Autodesk Inventor part; units mm, degrees
ref_plane "YZ Plane" through (0, 0, 0) normal (1, 0, 0) x (0, 1, 0)
ref_plane "XZ Plane" through (0, 0, 0) normal (0, 1, 0) x (-1, 0, 0)
ref_plane "XY Plane" through (0, 0, 0) normal (0, 0, 1) x (1, 0, 0)
sketch "Esquisse1" plane through (0, 0, 0) normal (1, 0, 0) x (0, 1, 0)
  line L0 (615.5373, -142.1522) -> (811.8285, -142.1522) construction
  line L1 (811.8285, -142.1522) -> (811.8285, -230.5611) construction
  line L2 (811.8285, -230.5611) -> (615.5373, -230.5611) construction
  line L3 (615.5373, -230.5611) -> (615.5373, -142.1522) construction
  circle A0 centre (714.0804, -164.9097) radius 9.3044
  circle A1 centre (714.0804, -164.9097) radius 12.8446
  arc A2 (718.2667, -201.6616) -> (719.1833, -202.8097) centre (719.23, -201.8325) ccw
  arc A3 (719.6606, -209.9141) -> (719.248, -210.7518) centre (719.7361, -210.4718) ccw
  arc A4 (713.6782, -215.3851) -> (712.2032, -215.3703) centre (712.9331, -216.1323) ccw
  line L4 (711.5826, -198.3788) -> (715.3474, -192.8257)
  line L5 (715.3474, -192.8257) -> (719.8038, -195.0511)
  line L6 (719.8038, -195.0511) -> (718.2667, -201.6616)
  line L7 (719.1833, -202.8097) -> (725.8864, -202.9912)
  line L8 (725.8864, -202.9912) -> (726.1597, -208.1294)
  line L9 (726.1597, -208.1294) -> (719.6606, -209.9141)
  line L10 (719.248, -210.7518) -> (722.051, -216.9958)
  line L11 (722.051, -216.9958) -> (717.7376, -219.4332)
  line L12 (717.7376, -219.4332) -> (713.6782, -215.3851)
  line L13 (712.2032, -215.3703) -> (708.5343, -221.0039)
  line L14 (708.5343, -221.0039) -> (704.0426, -218.7609)
  line L15 (704.0426, -218.7609) -> (705.4927, -212.5247)
  line L16 (704.6548, -211.4369) -> (698.081, -211.076)
  line L17 (698.081, -211.076) -> (698.1175, -205.8223)
  line L18 (698.1175, -205.8223) -> (703.9597, -204.218)
  line L19 (704.461, -202.9923) -> (701.4433, -196.9238)
  line L20 (701.4433, -196.9238) -> (705.5988, -194.2119)
  line L21 (705.5988, -194.2119) -> (709.8549, -198.4562)
  arc A5 (719.8038, -195.0511) -> (715.3474, -192.8257) centre (717.4272, -194.2357) ccw
  arc A6 (726.1597, -208.1294) -> (725.8864, -202.9912) centre (725.4624, -205.5902) ccw
  arc A7 (717.7376, -219.4332) -> (722.051, -216.9958) centre (719.7814, -218.0147) ccw
  arc A8 (704.0426, -218.7609) -> (708.5343, -221.0039) centre (706.417, -219.625) ccw
  arc A9 (698.1175, -205.8223) -> (698.081, -211.076) centre (698.2252, -208.45) ccw
  arc A10 (705.5988, -194.2119) -> (701.4433, -196.9238) centre (703.68, -195.8115) ccw
  arc A11 (709.8549, -198.4562) -> (711.5826, -198.3788) centre (710.6833, -197.6255) ccw
  arc A12 (703.9597, -204.218) -> (704.461, -202.9923) centre (703.6717, -203.3848) ccw
  arc A13 (705.4927, -212.5247) -> (704.6548, -211.4369) centre (704.6286, -212.3238) ccw
  point P0 (0, 0)
extrude "Extrusion1" add sketch "Esquisse1" against normal blind 3 contours A2 L7 L8 L9 A3 L10 L11 L12 A4 L13 L14 L15 A13 L16 L17 L18 A12 L19 L20 L21 A11 L4 L5 L6 | L5 A5 | A6 L8 | L20 A10 | A7 L11 | L17 A9 | A8 L14
sketch "Esquisse17" plane through (-3, 0, 0) normal (-1, 0, 0) x (0, 0, 1)
  circle A0 centre (-207.1899, 711.5984) radius 2.5
  point P0 (0, 0)
  dimension "d66" = 5
extrude "Extrusion11" cut sketch "Esquisse17" against normal blind 10
sketch "Esquisse18" plane through (-3, 0, 0) normal (-1, 0, 0) x (0, 0, 1)
  circle A0 centre (-207.1899, 711.5984) radius 2.5
  line L0 (-208.7203, 700.3139) -> (-205.4181, 706.7422)
  line L1 (-205.4181, 706.7422) -> (-197.0964, 704.8049)
  line L2 (-197.0964, 704.8049) -> (-202.9234, 711.5984)
  line L3 (-202.9234, 711.5984) -> (-197.0964, 716.5964)
  line L4 (-197.0964, 716.5964) -> (-204.6899, 715.7243)
  line L5 (-204.6899, 715.7243) -> (-205.9905, 723.6937)
  line L6 (-205.9905, 723.6937) -> (-208.7203, 716.5964)
  line L7 (-208.7203, 716.5964) -> (-216.1173, 718.7623)
  line L8 (-216.1173, 718.7623) -> (-212.4188, 712.8623)
  line L9 (-212.4188, 712.8623) -> (-217.8785, 707.1825)
  line L10 (-217.8785, 707.1825) -> (-210.6003, 707.9486)
  line L11 (-210.6003, 707.9486) -> (-208.7203, 700.3139)
  circle A1 centre (-207.1899, 711.5984) radius 19.7592
  point P0 (0, 0)
extrude "Extrusion12" cut sketch "Esquisse18" against normal blind 10 contours A1
properties part number "palonnier"
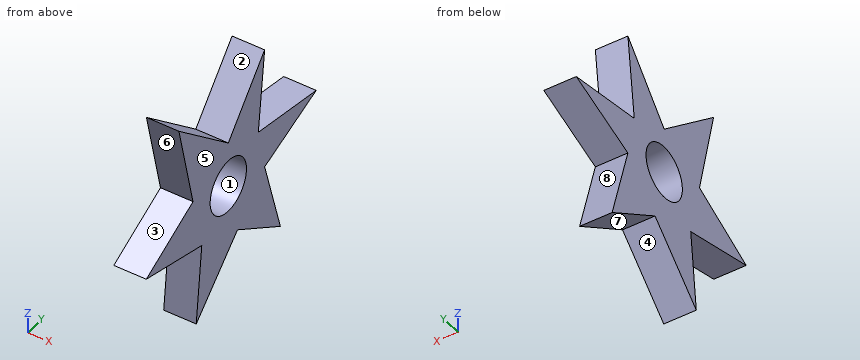
For this review, take the finished solid that the model builds, in its own axes (mm). Face numbers are marked on the shaded views. A direction names the side the tool comes from. Coordinates: 2 decimals unless noted, no trailing zeros. Order: outer loops, then holes, each group sorted by start corner. A loop starts at its lowest first (then second) coordinate and runs counter-clockwise, first axis right, second up. Notation, with made-up numbers: (-21, -21) -> (10, -21) arc R26 ccw to (10, 15) -> close; hole circle Ø6 at (-31, -38.75). An arc over 180 degrees is marked (long way). Return JSON: item names as keys, results as strings.
1. For pin 1 Ø1.5 at (x, z) = (-2, -211.5) entering from -Y, flat-tipped, find the tip position at first contact; note if it passes through.
Answer block:
{"pin 1": "y = 707.77"}
2. We need section D-D on y = 702.25. Write out the cut boundary in (x, z).
Answer block:
{"outline": "(-3, -209.2) -> (0, -209.2) -> (0, -207.73) -> (-3, -207.73) -> close"}
3. We need section B-B on y = 707.5. Write out the cut boundary in (x, z).
Answer block:
{"outline": "(-3, -217.57) -> (0, -217.57) -> (0, -214.86) -> (-3, -214.86) -> close; (-3, -210.49) -> (0, -210.49) -> (0, -199.41) -> (-3, -199.41) -> close"}
4. The part is to be moulded in two halves that separate along Z. For the marked faces 1, 2, 3 and 4, say which applies: +Z half, -Z half, draft (parallel to the pull), parting line (faces both ways), or undercut.
Answer block:
{"face 1": "undercut", "face 2": "+Z half", "face 3": "undercut", "face 4": "-Z half"}
5. Machinability: for the marked faces 5, 6, 7 and 8, which of the approach directions +Z, -Z, +X, -X, +Y, -Y give a long, thin tool a straight path to every point of the face, cutting with its end or side? Answer none if there is none.
Answer block:
{"face 5": "+Z, -Z, +X, +Y, -Y", "face 6": "+X, -X, -Y", "face 7": "-Z, +X, -X", "face 8": "+X, -X, +Y"}
6. For line 1 (Y direction, x = -1.85, z = -199.5); line 2 (Y direction, x = -0.35, z = -202.5); line 3 (Z direction, x = -0.15, y = 710), list the stretches that pass through material, from the lowest coordinate up. Write a range as from..to.
Answer block:
{"line 1": "705.36..707.61, 714.53..716.32", "line 2": "706.06..711.1, 711.96..715.98", "line 3": "-215.17..-209.11, -205.27..-201.55"}
7. We need section C-C on z = -200. Write out the cut boundary in (x, y).
Answer block:
{"outline": "(-3, 705.48) -> (0, 705.48) -> (0, 708.19) -> (-3, 708.19) -> close; (-3, 714.11) -> (0, 714.11) -> (0, 716.26) -> (-3, 716.26) -> close"}
8. We need section A-A on x = -0.85. Write out the cut boundary in (y, z), and give its area (3 significant figures).
Answer block:
{"outline": "(700.31, -208.72) -> (707.95, -210.6) -> (707.18, -217.88) -> (712.86, -212.42) -> (718.76, -216.12) -> (716.6, -208.72) -> (723.69, -205.99) -> (715.72, -204.69) -> (716.6, -197.1) -> (711.6, -202.92) -> (704.8, -197.1) -> (706.74, -205.42) -> close; hole circle Ø5 at (711.6, -207.19)", "area": "154 mm²"}
